from build123d import *

# Parameters (mm, degrees)
F1_DEPTH = 160
F3_D     = 5
F3_DEPTH = 5
F3_TIP   = 1.5021515476
F4_W     = 8.2
F4_H     = 5.2
F5_DEPTH = 11
F7_D     = 3
F6_W     = 4
F6_H     = 3
F8_DEPTH = 1
F9_R     = 2
F10_R    = 0.5


# Not quite as in the source:
# - a feature names something its author has since deleted; it is built from what else it names


with BuildPart() as f1:
    # F0 (on Right) → F1 (new body)
    with BuildSketch(Plane.YZ):
        Polygon((9.9597979746, -9.0402020254), (12, -7), (12, 0), (0, 0), (0, -6.5), (0, -19), (3.4544155877, -15.5455844123), (2.7473088065, -14.8384776311), (9.2526911935, -8.3330952442), align=None)
    extrude(amount=F1_DEPTH)

    # F3
    with Locations(Plane.XY):
        with Locations((90, 6), (70, 6)):
            Hole(F3_D / 2, depth=F3_DEPTH)
            with Locations((0, 0, -(F3_DEPTH + F3_TIP / 2))):  # 118° drill point
                Cone(0, F3_D / 2, F3_TIP, mode=Mode.SUBTRACT)

    # F4 (on face) → F5 (cut)
    with BuildSketch(Plane(origin=(0, 12, 0), x_dir=(-1, 0, 0), z_dir=(0, 1, 0))):
        with Locations((-90, -3.6)):
            Rectangle(F4_W, F4_H)
        with Locations((-70, -3.6)):
            Rectangle(F4_W, F4_H)
    extrude(amount=-F5_DEPTH, mode=Mode.SUBTRACT)

    # F7 (through all)
    with Locations(Plane.XY):
        with Locations((4, 6), (156, 6)):
            Hole(F7_D / 2)

    # F6 (on Top) → F8 (cut)
    with BuildSketch(Plane.XY):
        with Locations((158, 6)):
            Rectangle(F6_W, F6_H)
        with Locations((2, 5.8232012801)):
            Rectangle(F6_W, F6_H)
    extrude(amount=-F8_DEPTH, mode=Mode.SUBTRACT)

    # F9
    f9_edges = [f1.edges().sort_by_distance(p)[0] for p in [
        (80, 0, -19),
    ]]
    fillet(f9_edges, radius=F9_R)

    # F10
    f10_edges = [f1.edges().sort_by_distance(p)[0] for p in [
        (160, 10.979899, -8.020101),
        (0, 10.979899, -8.020101),
        (160, 3.434315, -15.565685),
        (0, 3.434315, -15.565685),
        (0, 1.234633, -16.019332),
        (0, 0, -7.085786),
        (160, 1.234633, -16.019332),
        (160, 0, -7.085786),
        (80, 9.959798, -9.040202),
        (80, 12, -7),
    ]]
    fillet(f10_edges, radius=F10_R)


solid = f1.part
Source: CAD feature listing. Evaluate the final solid. Frame: model axes, mm. A direction names the side the tool comes from. Give positions to 0.01 mm unless a question says otherwise; leave off trailing zeros. Write each loop counter-clockwise with the first axis right and the second up, starting at its lowest first coordinate (ties: lowest second). Pieces come first, ordered by that corner, then holes. Notation, with made-up numbers: (-11, 0) -> (0, 0) arc R24 cw to (0, 14) -> close; hole circle Ø9 at (8, -24). An arc over 180 degrees is marked (long way). Return JSON: item names as keys, results as strings. Group by question number.
1. Access query for faces 4 (the face through (92.5, 6.1, -0.5)), 5 (the face through (158, 6, -1)), 6 (the face through (65.9, 7, -4)). Directions: +Z, -Z, +X, -X, +Y, -Y. A direction counts if a zero-diameter tool reaches every point of the face in a straight line with its end or side. Return the directions, or none.
2. Material intervals for line 1 (X direction, y = 9.5, z = -5); line 2 (Z direction, x = 86, y = 10); line 3 (Y direction, x = 4, z = -4.25), sorted ascending. Write a range as from..to.
3. Pin query (flat end, axial travel): pin 1 Ø2.5 at (x, y) = (69.5, 8) entering from -Z; pin 2 Ø4 at (x, y) = (51, 2.5) entering from -Z; pin 3 Ø4.5 at (x, y) = (70, 6) entering from -Z; pin 4 Ø1.6 at (x, z) = (88, -4) entering from +Y. Return the tip coordinate at first contact, or that it passes through.
4. Section B-B, the plane x = 139.5. Output: boundary loops of the cut face in (y, z), then the cut area to 3 significant figures.
5. Mould query, pull axis X, two halves, no side actions, for faces 1 (the face through (79, 12, -3)), 2 (the face through (72.5, 6.1, -0.5)), 3 (the face through (160, 5, -6)). Classes: +X half, -X half, draft (parallel to the pull), parting line (faces both ways), or undercut.
6. Section A-A, the plane z = -3.5. Output: boundary loops of the cut face in (x, y), then the cut area to 3 significant figures.
Determined:
{
 "1": {"face 4": "+Z", "face 5": "+Z, +X", "face 6": "+Y"},
 "2": {"line 1": "x = 0..65.9, 74.1..85.9, 94.1..160", "line 2": "z = -8.83..-6.2, -1..0", "line 3": "y = 0..4.5, 7.5..12"},
 "3": {"pin 1": "stops at z = -10.84", "pin 2": "stops at z = -16.17", "pin 3": "stops at z = -13.84", "pin 4": "stops at y = 1"},
 "4": {"outline": "(0, -14.17) arc R2 ccw to (3.41, -15.59) -> (3.45, -15.55) -> (2.75, -14.84) -> (9.25, -8.33) -> (9.61, -8.69) arc R0.5 ccw to (10.31, -8.69) -> (11.85, -7.15) arc R0.5 ccw to (12, -6.79) -> (12, 0) -> (0, 0) -> close", "area": "142 mm2"},
 "5": {"face 1": "draft", "face 2": "undercut", "face 3": "+X half"},
 "6": {"outline": "(0, 0.5) arc R0.5 ccw to (0.5, 0) -> (159.5, 0) arc R0.5 ccw to (160, 0.5) -> (160, 12) -> (94.1, 12) -> (94.1, 1) -> (85.9, 1) -> (85.9, 12) -> (74.1, 12) -> (74.1, 1) -> (65.9, 1) -> (65.9, 12) -> (0, 12) -> close; hole circle Ø3 at (4, 6); hole circle Ø3 at (156, 6)", "area": "1,730 mm2"}
}
